Build history of the part. All positions in model axes, mm. A direction names the side the tool comes from. Round coordinates to 2 decimals unless told otherwise and drop trailing zeros. Write each loop counter-clockwise with the first axis right and the second up, starting at its lowest first coordinate (ties: lowest second). Pieces come first, ordered by that corner, then holes. Notation, with made-up numbers: (-30, 40) -> (-13, 40) arc R8 cw to (-13, 46) -> close; hole circle Ø5 at (84, 80). An arc over 180 degrees is marked (long way). One line per question, with ' | ' between items.
from build123d import *

# Parameters (mm, degrees)
SKETCH1_W              = 100
SKETCH1_H              = 100
BOSS_EXTRUDE1_DEPTH    = 6
SKETCH234_W            = 6
SKETCH234_H            = 6
BOSS_EXTRUDE234_DEPTH  = 6
FILLET134_R            = 1
SKETCH2342_W           = 10
SKETCH2342_H           = 6
BOSS_EXTRUDE2342_DEPTH = 6
FILLET1342_R           = 1


with BuildPart() as part:
    # Sketch1 → Boss-Extrude1 (new body)
    with BuildSketch(Plane(origin=(0, 0, 0), x_dir=(1, 0, 0), z_dir=(0, 1, 0))):
        Rectangle(SKETCH1_W, SKETCH1_H)
    extrude(amount=BOSS_EXTRUDE1_DEPTH)

    # Sketch234 → Boss-Extrude234 (add)
    with BuildSketch(Plane.XY.offset(50)):
        with Locations((0.767778608, 3)):
            Rectangle(SKETCH234_W, SKETCH234_H)
    extrude(amount=BOSS_EXTRUDE234_DEPTH)

    # Fillet134
    fillet134_edges = [part.edges().sort_by_distance(p)[0] for p in [
        (-2.232221392, 3, 56),
        (3.767778608, 3, 56),
    ]]
    fillet(fillet134_edges, radius=FILLET134_R)

    # Sketch2342 → Boss-Extrude2342 (add)
    with BuildSketch(Plane(origin=(-28.445435161, 6, 50), x_dir=(-1, 0, 0), z_dir=(0, 0, 1))):
        with Locations((0.767778608, 3)):
            Rectangle(SKETCH2342_W, SKETCH2342_H)
    extrude(amount=BOSS_EXTRUDE2342_DEPTH)

    # Fillet1342
    fillet1342_edges = [part.edges().sort_by_distance(p)[0] for p in [
        (-34.213213769, 3, 56),
        (-24.213213769, 3, 56),
    ]]
    fillet(fillet1342_edges, radius=FILLET1342_R)


solid = part.part
(1) Wall check: line 1 (X direction, y = 3.1, z = 50.5); line 2 (Z direction, x = -17.5, y = 1.4). Give the ranges that are in metal, low to high. Write a range as from..to.
Calculated:
line 1: -34.21..-24.21, -2.23..3.77 | line 2: -50..50
(2) 3-axis set-ups, long thin cutter, end or side, ignore diameter. For faces 5 (the flat face through (1, 3, 56)), 6 (the flat face through (-34.213, 3, 52)), 7 (the flat face through (-24.213, 3, 52)), 8 (the flat face through (27, 3, 50)), 9 (the flat face through (-1, 3, -50)): which of +Z, -Z, +X, -X, +Y, -Y reach the whole face in a straight line?
Calculated:
face 5: +Z, +X, -X, +Y, -Y | face 6: +Z, -X, +Y, -Y | face 7: +Z, +Y, -Y | face 8: +Z, +X, +Y, -Y | face 9: -Z, +X, -X, +Y, -Y
(3) Slice it at A-A (y = 2). Write the cut outline in (x, z), then the cut area to 3 significant figures.
Calculated:
outline: (-50, -50) -> (50, -50) -> (50, 50) -> (3.77, 50) -> (3.77, 55) arc R1 ccw to (2.77, 56) -> (-1.23, 56) arc R1 ccw to (-2.23, 55) -> (-2.23, 50) -> (-24.21, 50) -> (-24.21, 55) arc R1 ccw to (-25.21, 56) -> (-33.21, 56) arc R1 ccw to (-34.21, 55) -> (-34.21, 50) -> (-50, 50) -> close | area: 10,100 mm2
(4) Slice it at B-B (x = -37.5). Write the cut outline in (y, z).
Calculated:
outline: (0, -50) -> (6, -50) -> (6, 50) -> (0, 50) -> close
(5) Drop flat-ended pins along their axis: pin 1 (1 mm diameter, centred on x = -37.5, z = 29, fed in from -Y); pin 2 (2.5 mm diameter, centred on y = 2.5, z = 53.5, fed in from +X); pin 3 (1.8 mm diameter, centred on x = -14, y = 4.5, fed in from +Z); pin 4 (2.5 mm diameter, centred on y = 2, z = 52.5, fed in from -X). Give the stop position or say it passes through.
Calculated:
pin 1: y = 0 | pin 2: x = 3.77 | pin 3: z = 50 | pin 4: x = -34.21
(6) Mould opens along X. For faces 1 (the flat face through (-42, 3, 50)), 2 (the flat face through (3.768, 3, 52)), 3 (the flat face through (-13, 3, 50)), 4 (the flat face through (-50, 3, 1)) say: pulls with the +X half, pulls with the -X half, needs draft (parallel to the pull), parting line crosses it, or undercut.
Calculated:
face 1: needs draft | face 2: pulls with the +X half | face 3: undercut | face 4: pulls with the -X half
